Verification items for the finished model (mm, model axes). A direction names the side the tool comes from. Coordinates: 2 decimals unless noted, no trailing zeros. Order: outer loops, then holes, each group sorted by start corner. A loop starts at its lowest first (then second) coordinate and runs counter-clockwise, first axis right, second up. Notation, with made-up numbers: M 55.25,-7 L 65.25,-7 A18 ccw 65.25,13 Z; hole C 65.5,25.25 d7. An arc over 180 degrees is marked long. Answer as a JSON object with one key per item and string values. Group by question number.
(1) Cross-section at D-D (z = -22). Enter the section's corners in (x, y).
(2) Access from +Z, -Z, +X, -X, +Y, -Y to the whole of each face (thin tool, end or side, straight path). Record for faces 4 (the face through (-20, 1, -6)), 5 (the face through (-6, 1, 20)), 6 (the face through (0, 2, 14)).
(3) Material ranges on line 1 (X direction, y = 2.6, z = 0); line 2 (Z direction, x = 26, y = 1), recorded low to high.
(4) Mould release check, pull along X, two halves, no side actions. Record for faces 1 (the face through (-20, 1, 6)), 2 (the face through (-0.195, 1.479, 24.513)), 3 (the face through (11.25, 1.232, 11.377)): released by +X, released by -X, zero draft, split by the parting line, or undercut.
(5) Cross-section at A-A (z = 0). Count the separate pieces of the cut face and the enclosed holes in it, plus the area to 3 significant figures.
(6) Cross-section at C-C (x = -23). Enter the section's corners in (y, z), plus the area to 3 significant figures.
(7) Gauge pin test, flat ends, axial feed: pin 1 Ø2 at (x, z) = (-21, -8.5) entering from -Y; pin 2 Ø1.5 at (y, z) = (1.5, 18) entering from -X; pin 3 Ø1.2 at (x, y) = (-20.5, 1.5) entering from -Z; pin 4 Ø0.8 at (y, z) = (1, 21.5) entering from +X. Record the tip position at first contact, or that the pin passes through.
from build123d import *

# Parameters (mm, degrees)
SKETCH1_R           = 6
SKETCH1_R_2         = 1.5
BOSS_EXTRUDE1_DEPTH = 3
FILLET1_R           = 0.5
SKETCH2_R           = 1.5
CUT_EXTRUDE1_DEPTH  = 4
CHAMFER1_SIZE       = 1.75


with BuildPart() as part:
    # Sketch1 → Boss-Extrude1 (new body)
    with BuildSketch(Plane(origin=(0, 0, 0), x_dir=(1, 0, 0), z_dir=(0, 1, 0))):
        with BuildLine():
            Line((26, 6), (14.832396974, 6))
            ThreePointArc((14.832396974, 6), (11.313708499, 11.313708499), (6, 14.832396974))
            Line((6, 14.832396974), (6, 26))
            ThreePointArc((6, 26), (0, 32), (-6, 26))
            Line((-6, 26), (-6, 14.832396974))
            ThreePointArc((-6, 14.832396974), (-11.313708499, 11.313708499), (-14.832396974, 6))
            Line((-14.832396974, 6), (-26, 6))
            ThreePointArc((-26, 6), (-32, 0), (-26, -6))
            Line((-26, -6), (-14.832396974, -6))
            ThreePointArc((-14.832396974, -6), (-11.313708499, -11.313708499), (-6, -14.832396974))
            Line((-6, -14.832396974), (-6, -26))
            ThreePointArc((-6, -26), (0, -32), (6, -26))
            Line((6, -26), (6, -14.832396974))
            ThreePointArc((6, -14.832396974), (11.313708499, -11.313708499), (14.832396974, -6))
            Line((14.832396974, -6), (26, -6))
            ThreePointArc((26, -6), (32, 0), (26, 6))
        make_face()
        Circle(SKETCH1_R, mode=Mode.SUBTRACT)
        with Locations((0, 26)):
            Circle(SKETCH1_R_2, mode=Mode.SUBTRACT)
        with Locations((26, 0)):
            Circle(SKETCH1_R_2, mode=Mode.SUBTRACT)
        with Locations((0, -26)):
            Circle(SKETCH1_R_2, mode=Mode.SUBTRACT)
        with Locations((-26, 0)):
            Circle(SKETCH1_R_2, mode=Mode.SUBTRACT)
    extrude(amount=BOSS_EXTRUDE1_DEPTH)

    # Fillet1
    fillet1_edges = [part.edges().sort_by_distance(p)[0] for p in [
        (-11.313708499, 3, -11.313708499),
        (-20.416198487, 3, -6),
        (-32, 3, 0),
        (-20.416198487, 3, 6),
        (-11.313708499, 3, 11.313708499),
        (-6, 3, 20.416198487),
        (0, 3, 32),
        (6, 3, 20.416198487),
        (11.313708499, 3, 11.313708499),
        (20.416198487, 3, 6),
        (0, 3, -32),
        (32, 3, 0),
        (20.416198487, 3, -6),
        (11.313708499, 3, -11.313708499),
        (6, 3, -20.416198487),
        (-6, 3, -20.416198487),
    ]]
    fillet(fillet1_edges, radius=FILLET1_R)

    # Sketch2 → Cut-Extrude1 (cut, through all)
    with BuildSketch(Plane(origin=(0, 3, 0), x_dir=(1, 0, 0), z_dir=(0, 1, 0))):
        with Locations((0, 12.5)):
            Circle(SKETCH2_R)
        with Locations((12.5, 0)):
            Circle(SKETCH2_R)
        with Locations((0, -12.5)):
            Circle(SKETCH2_R)
        with Locations((-12.5, 0)):
            Circle(SKETCH2_R)
    extrude(amount=-CUT_EXTRUDE1_DEPTH, mode=Mode.SUBTRACT)

    # Chamfer1
    chamfer1_edges = [part.edges().sort_by_distance(p)[0] for p in [
        (-1.5, 0, -12.5),
        (11, 0, 0),
        (-1.5, 0, 12.5),
        (-14, 0, 0),
    ]]
    chamfer(chamfer1_edges, length=CHAMFER1_SIZE)


solid = part.part
Taken from the geometry:
{
 "1": {"outline": "M -6,0 L 6,0 L 6,2.5 A0.5 ccw 5.5,3 L -5.5,3 A0.5 ccw -6,2.5 Z"},
 "2": {"face 4": "-Z, -X, +Y, -Y", "face 5": "+Z, -X, +Y, -Y", "face 6": "+Y, -Y"},
 "3": {"line 1": "x = -31.99 to -27.5, -24.5 to -14, -11 to -6, 6 to 11, 14 to 24.5, 27.5 to 31.99", "line 2": "z = -6 to -1.5, 1.5 to 6"},
 "4": {"face 1": "zero draft", "face 2": "undercut", "face 3": "released by +X"},
 "5": {"separate pieces": "6", "enclosed holes": "0", "area": "114 mm²"},
 "6": {"outline": "M 0,-6 L 2.5,-6 A0.5 ccw 3,-5.5 L 3,5.5 A0.5 ccw 2.5,6 L 0,6 Z", "area": "35.9 mm²"},
 "7": {"pin 1": "passes through", "pin 2": "stops at x = -6", "pin 3": "stops at z = -6", "pin 4": "stops at x = 6"}
}
